Could you check a few things on this model? Use its own coordinates, in mm. A direction names the side the tool comes from. Coordinates: 2 decimals unless noted, no trailing zeros. Write each loop counter-clockwise with the first axis right and the second up, starting at its lowest first coordinate (ties: lowest second). Pieces come first, ordered by that corner, then holes.
Item 1: Thinking about a two-plate mould opening in Y: for faces 3 (the flat face through (23.277, -50.857, 9.747)), 4 (the flat face through (11.062, 54.826, 9.747)), 5 (the flat face through (28.3, 16.945, 12.522)), which applies, +Y half, -Y half, draft (parallel to the pull), parting line (faces both ways), or undercut?
Item 2: For P1, Ø14.5, axis at x = -26.5, y = 26.5, coming from the +Z side; P2, Ø4, axis at x = -43.5, z = 17.5, coming from the -Y side; P3, Ø3, axis at x = -33.5, z = 14.5, coming from the -Y side; P4, Ø5, axis at x = -3, z = 19, coming from the -Y side, each with a flat end and sliding along its axis, tell me the tip position at first contact or that it passes through.
Item 3: I want a section at B-B on x = 6. Please give me the cut outline in (y, z), then the cut area to 3 significant figures.
Item 4: Which directions (+Z, -Z, +X, -X, +Y, -Y) give clear straight access to the entire face, cutting with the end or side of a thin tool? Please do faces 1 (the flat face through (20.53, -45.13, 12.52)), 2 (the flat face through (-48.724, 27.463, 9.747)).
Item 5: I want a section at C-C on y = 40.5. Please give me the cut outline in (x, z), then the cut area to 3 significant figures.
Item 6: If I drill on probe 1 along Y at (x, z) = (19.5, 21); probe 2 along Y at (x, z) = (-29.5, 11); probe 3 along Y at (x, z) = (-32, 18), over which ranges is the centre line in solid material (lowest first)?
Item 7: I want a section at A-A on z = 23.5. Please give me the cut outline in (x, y), then the cut area to 3 significant figures.
Item 8: I want a section at D-D on x = 33. Please give me the cut outline in (y, z).
from build123d import *

# Parameters (mm, degrees)
F1_DEPTH = 25.4
F2_DEPTH = 25.4
F4_DEPTH = 6.35


with BuildPart() as f1:
    # F0 (on Top) → F1 (new body)
    with BuildSketch(Plane.XY):
        Polygon((0, 0), (-14.361076, -67.622363), (59.874873, -34.554655), align=None)
        Polygon((4.395829, -9.868497), (45.906835, -33.825098), (-5.560647, -56.750806), align=None, mode=Mode.SUBTRACT)
        Polygon((0, 0), (-68.750506, -7.238264), (-14.361076, -67.622363), align=None)
        Polygon((-17.983588, -54.112525), (-55.691559, -12.248475), (-8.027112, -7.230215), align=None, mode=Mode.SUBTRACT)
        Polygon((51.365783, 46.266412), (-28.129073, 63.14887), (0, 0), align=None)
        Polygon((-17.257516, 54.34844), (37.855945, 42.643901), (2.244256, 10.567585), align=None, mode=Mode.SUBTRACT)
        Polygon((51.365783, 46.266412), (0, 0), (59.874873, -34.554655), align=None)
        Polygon((46.355573, 33.207464), (52.25489, -22.825453), (10.743884, 1.131149), align=None, mode=Mode.SUBTRACT)
    extrude(amount=F1_DEPTH)

    # F0 (on Top) → F2 (join)
    with BuildSketch(Plane.XY):
        Polygon((0, 0), (-68.750506, -7.238264), (-14.361076, -67.622363), align=None)
        Polygon((-17.983588, -54.112525), (-55.691559, -12.248475), (-8.027112, -7.230215), align=None, mode=Mode.SUBTRACT)
        Polygon((-28.129073, 63.14887), (-68.750506, -7.238264), (0, 0), align=None)
        Polygon((-57.021304, 0.381718), (-28.85863, 49.180833), (-9.356857, 5.399978), align=None, mode=Mode.SUBTRACT)
        Polygon((51.365783, 46.266412), (-28.129073, 63.14887), (0, 0), align=None)
        Polygon((-17.257516, 54.34844), (37.855945, 42.643901), (2.244256, 10.567585), align=None, mode=Mode.SUBTRACT)
        Polygon((0, 0), (-14.361076, -67.622363), (59.874873, -34.554655), align=None)
        Polygon((4.395829, -9.868497), (45.906835, -33.825098), (-5.560647, -56.750806), align=None, mode=Mode.SUBTRACT)
        Polygon((51.365783, 46.266412), (0, 0), (59.874873, -34.554655), align=None)
        Polygon((46.355573, 33.207464), (52.25489, -22.825453), (10.743884, 1.131149), align=None, mode=Mode.SUBTRACT)
    extrude(amount=F2_DEPTH)

    # F3 (on face) → F4 (join)
    with BuildSketch(Plane(origin=(0, 0, 0), x_dir=(1, 0, 0), z_dir=(0, 0, -1))):
        Polygon((-68.750506, 7.238264), (-28.129073, -63.14887), (51.365783, -46.266412), (59.874873, 34.554655), (-14.361076, 67.622363), align=None)
    extrude(amount=F4_DEPTH)


solid = f1.part
Response values:
1. face 3: -Y half
1. face 4: +Y half
1. face 5: undercut
2. P1: stops at z = 25.4
2. P2: stops at y = -37.49
2. P3: stops at y = -48.04
2. P4: stops at y = -63.68
3. outline: (-58.55, -6.35) - (55.9, -6.35) - (55.9, 25.4) - (49.41, 25.4) - (49.41, 0) - (13.95, 0) - (13.95, 25.4) - (-10.79, 25.4) - (-10.79, 0) - (-51.6, 0) - (-51.6, 25.4) - (-58.55, 25.4) - close
3. area: 1,700 mm2
4. face 1: +Z
4. face 2: +Z, -Z, -X, +Y
5. outline: (-41.2, -6.35) - (51.97, -6.35) - (51.97, 25.4) - (35.48, 25.4) - (35.48, 0) - (-11.09, 0) - (-11.09, 25.4) - (-24.99, 25.4) - (-24.99, 0) - (-33.87, 0) - (-33.87, 25.4) - (-41.2, 25.4) - close
5. area: 1,550 mm2
6. probe 1: y = -52.54 to -45.59, -18.59 to -3.92, 9.02 to 26.11, 46.54 to 53.03
6. probe 2: y = -50.81 to -41.33, -9.49 to 3.28, 48.07 to 60.77
6. probe 3: y = -48.04 to -38.55, -9.75 to 3.02, 43.74 to 56.44
7. outline: (-68.75, -7.24) - (-14.36, -67.62) - (59.87, -34.55) - (51.37, 46.27) - (-28.13, 63.15) - close; hole (-57.02, 0.38) - (-9.36, 5.4) - (-28.86, 49.18) - close; hole (-55.69, -12.25) - (-17.98, -54.11) - (-8.03, -7.23) - close; hole (-17.26, 54.35) - (2.24, 10.57) - (37.86, 42.64) - close; hole (-5.56, -56.75) - (45.91, -33.83) - (4.4, -9.87) - close; hole (10.74, 1.13) - (52.25, -22.83) - (46.36, 33.21) - close
7. area: 5,900 mm2
8. outline: (-46.53, -6.35) - (50.17, -6.35) - (50.17, 25.4) - (43.68, 25.4) - (43.68, 0) - (38.27, 0) - (38.27, 25.4) - (21.18, 25.4) - (21.18, 0) - (-11.71, 0) - (-11.71, 25.4) - (-26.38, 25.4) - (-26.38, 0) - (-39.57, 0) - (-39.57, 25.4) - (-46.53, 25.4) - close
